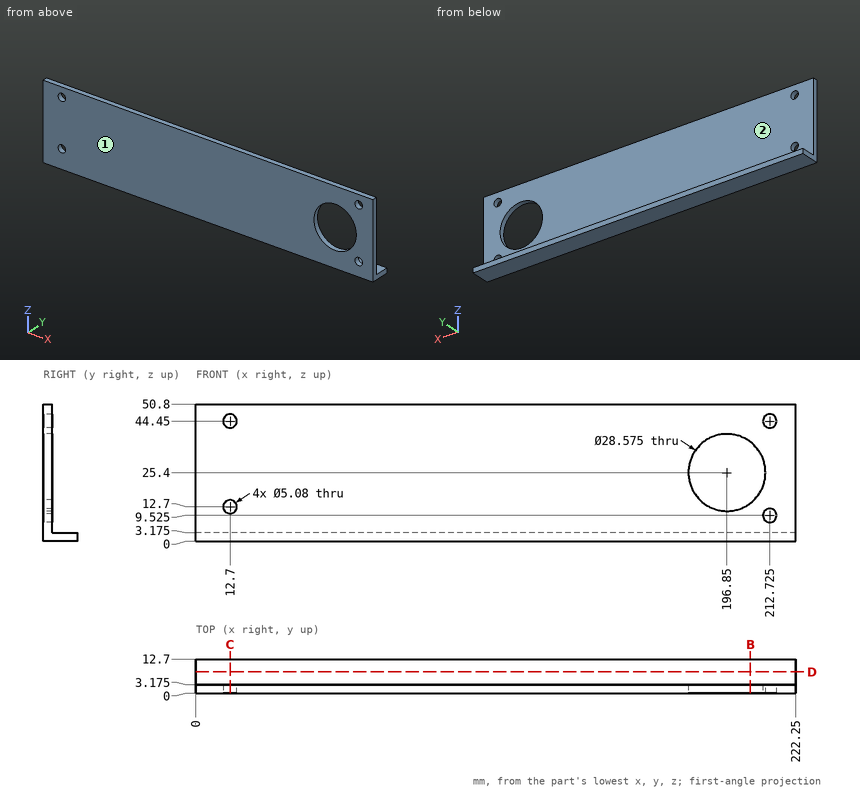
Verification items for this drawing (mm, ordinates from the low corner). A direction names the side the tool comes from. Give positions to 0.01 mm unless a question says otherwise; leave off trailing zeros. Write each loop counter-clockwise with the first axis right and the second up, starting at its lowest first coordinate (ties: lowest second). Pieces come first, ordered by that corner, then holes. Notation, with made-up numbers: (19, -35.75) - (35, -35.75) arc R13 ccw to (35, -30.75) - close; hole circle Ø3 at (-37.5, 38). An arc over 180 degrees is marked (long way). Answer as a JSON object with one key per item and string values. Group by question number.
1) Access from +Z, -Z, +X, -X, +Y, -Y to the whole of each face (thin tool, end or side, straight path). Record for the marked faces 1 and 2.
2) Depth check by flat-ended pin: P1, Ø12, axis at x = 119, z = 31, coming from the +Y side (3 decimals); P2, Ø5, axis at x = 126, y = 6, coming from the +Z side (3 decimals). Enter the tip coordinate at first touch or a pass-through.
3) Sectioned sample at C-C (x = 12.7). Record the cut outline in (y, z) (3 decimals).
4) Thickness scan on probe 1 along Z at (x, y) = (12.7, 2.55); probe 2 along Z at (x, y) = (65, 10.75) (3 decimals). Record the ranges inside material, lowest first. Write a range as from..to.
5) Sectioned sample at B-B (x = 205.5). Record the cut outline in (y, z) (3 decimals), then the cut area to 3 significant figures.
6) Sectioned sample at D-D (y = 8). Record the cut outline in (x, z) (3 decimals).
Geometry results:
{
 "1": {"face 1": "+Z, -Z, +X, -X, -Y", "face 2": "+Z, +X, -X, +Y"},
 "2": {"P1": "stops at y = 3.175", "P2": "stops at z = 3.175"},
 "3": {"outline": "(0, 0) - (12.7, 0) - (12.7, 3.175) - (3.175, 3.175) - (3.175, 10.16) - (0, 10.16) - close; (0, 15.24) - (3.175, 15.24) - (3.175, 41.91) - (0, 41.91) - close; (0, 46.99) - (3.175, 46.99) - (3.175, 50.8) - (0, 50.8) - close"},
 "4": {"probe 1": "z = 0..10.16, 15.24..41.91, 46.99..50.8", "probe 2": "z = 0..3.175"},
 "5": {"outline": "(0, 0) - (12.7, 0) - (12.7, 3.175) - (3.175, 3.175) - (3.175, 14.029) - (0, 14.029) - close; (0, 36.771) - (3.175, 36.771) - (3.175, 50.8) - (0, 50.8) - close", "area": "119 mm^2"},
 "6": {"outline": "(0, 0) - (222.25, 0) - (222.25, 3.175) - (0, 3.175) - close"}
}
